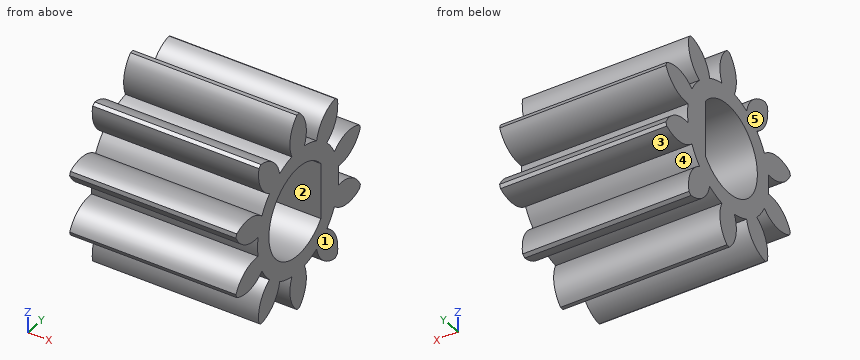
from build123d import *

# Parameters (mm, degrees)
SPUR_START             = -9.526796012
SPUR_GEAR_AM_OUTLINE_R = 2.5
SPUR_GEAR_AM_DEPTH     = 10
SKETCH1_R              = 2.7
CUT_EXTRUDE1_DEPTH     = 14.319939227
BOSS_EXTRUDE1_DEPTH    = 10


# Read off the part's stored shape, not the designer's step: spur gear_am
with BuildPart() as part:
    # spur gear_am outline → spur gear_am (new body)
    with BuildSketch(Plane.YZ.offset(SPUR_START)):
        with BuildLine():
            ThreePointArc((-0.156519062, -5.364277595), (-0.037626451, -5.365455666), (0.081266159, -5.364277595))
            ThreePointArc((0.081266159, -5.364277595), (0.682735226, -4.291319539), (0.542534544, -3.069293435))
            ThreePointArc((0.542534544, -3.069293435), (1.12087826, -2.930966545), (1.670074661, -2.702933442))
            ThreePointArc((1.670074661, -2.702933442), (2.274938849, -3.773981221), (3.392206468, -4.288487876))
            ThreePointArc((3.392206468, -4.288487876), (3.489085062, -4.219557632), (3.584578752, -4.14872123))
            ThreePointArc((3.584578752, -4.14872123), (3.440508527, -2.927145281), (2.608794871, -2.020913288))
            ThreePointArc((2.608794871, -2.020913288), (2.995378261, -1.569062577), (3.305652987, -1.061770376))
            ThreePointArc((3.305652987, -1.061770376), (4.424544483, -1.572735982), (5.630852398, -1.33226718))
            ThreePointArc((5.630852398, -1.33226718), (5.668712646, -1.219557632), (5.704332072, -1.106119996))
            ThreePointArc((5.704332072, -1.106119996), (4.869752484, -0.202526647), (3.664212201, 0.041761415))
            ThreePointArc((3.664212201, 0.041761415), (3.711373549, 0.634544334), (3.664212201, 1.227327254))
            ThreePointArc((3.664212201, 1.227327254), (4.869752484, 1.471615316), (5.704332072, 2.375208665))
            ThreePointArc((5.704332072, 2.375208665), (5.668712646, 2.488646301), (5.630852398, 2.601355849))
            ThreePointArc((5.630852398, 2.601355849), (4.424544483, 2.84182465), (3.305652987, 2.330859045))
            ThreePointArc((3.305652987, 2.330859045), (2.995378261, 2.838151246), (2.608794871, 3.290001957))
            ThreePointArc((2.608794871, 3.290001957), (3.440508527, 4.19623395), (3.584578752, 5.417809899))
            ThreePointArc((3.584578752, 5.417809899), (3.489085062, 5.488646301), (3.392206468, 5.557576545))
            ThreePointArc((3.392206468, 5.557576545), (2.274938849, 5.04306989), (1.670074661, 3.972022111))
            ThreePointArc((1.670074661, 3.972022111), (1.12087826, 4.200055214), (0.542534544, 4.338382103))
            ThreePointArc((0.542534544, 4.338382103), (0.682735226, 5.560408207), (0.081266159, 6.633366264))
            ThreePointArc((0.081266159, 6.633366264), (-0.037626451, 6.634544334), (-0.156519062, 6.633366264))
            ThreePointArc((-0.156519062, 6.633366264), (-0.757988129, 5.560408207), (-0.617787447, 4.338382103))
            ThreePointArc((-0.617787447, 4.338382103), (-1.196131163, 4.200055214), (-1.745327564, 3.972022111))
            ThreePointArc((-1.745327564, 3.972022111), (-2.350191752, 5.04306989), (-3.467459371, 5.557576545))
            ThreePointArc((-3.467459371, 5.557576545), (-3.564337965, 5.488646301), (-3.659831655, 5.417809899))
            ThreePointArc((-3.659831655, 5.417809899), (-3.51576143, 4.19623395), (-2.684047774, 3.290001957))
            ThreePointArc((-2.684047774, 3.290001957), (-3.070631163, 2.838151245), (-3.38090589, 2.330859045))
            ThreePointArc((-3.38090589, 2.330859045), (-4.499797386, 2.84182465), (-5.706105301, 2.601355849))
            ThreePointArc((-5.706105301, 2.601355849), (-5.743965549, 2.488646301), (-5.779584975, 2.375208665))
            ThreePointArc((-5.779584975, 2.375208665), (-4.945005387, 1.471615316), (-3.739465104, 1.227327254))
            ThreePointArc((-3.739465104, 1.227327254), (-3.786626451, 0.634544334), (-3.739465104, 0.041761415))
            ThreePointArc((-3.739465104, 0.041761415), (-4.945005387, -0.202526647), (-5.779584975, -1.106119996))
            ThreePointArc((-5.779584975, -1.106119996), (-5.743965549, -1.219557632), (-5.706105301, -1.33226718))
            ThreePointArc((-5.706105301, -1.33226718), (-4.499797386, -1.572735982), (-3.38090589, -1.061770376))
            ThreePointArc((-3.38090589, -1.061770376), (-3.070631163, -1.569062576), (-2.684047774, -2.020913288))
            ThreePointArc((-2.684047774, -2.020913288), (-3.51576143, -2.927145281), (-3.659831655, -4.14872123))
            ThreePointArc((-3.659831655, -4.14872123), (-3.564337965, -4.219557632), (-3.467459371, -4.288487876))
            ThreePointArc((-3.467459371, -4.288487876), (-2.350191752, -3.773981221), (-1.745327564, -2.702933442))
            ThreePointArc((-1.745327564, -2.702933442), (-1.196131163, -2.930966545), (-0.617787447, -3.069293435))
            ThreePointArc((-0.617787447, -3.069293435), (-0.757988129, -4.291319539), (-0.156519062, -5.364277595))
        make_face()
        with Locations((-0.037626451, 0.634544334)):
            Circle(SPUR_GEAR_AM_OUTLINE_R, mode=Mode.SUBTRACT)
    extrude(amount=SPUR_GEAR_AM_DEPTH)

    # Sketch1 → Cut-Extrude1 (cut, through all)
    with BuildSketch(Plane.ZY.offset(9.526796012)):
        with Locations((0.634544334, -0.037626451)):
            Circle(SKETCH1_R)
    extrude(amount=-CUT_EXTRUDE1_DEPTH, mode=Mode.SUBTRACT)

    # Sketch2 → Boss-Extrude1 (add, through all)
    with BuildSketch(Plane.ZY.offset(9.526796012)):
        with BuildLine():
            Line((2.331600609, 2.062373549), (-1.06251194, 2.062373549))
            ThreePointArc((-1.06251194, 2.062373549), (0.634544334, 2.662373549), (2.331600609, 2.062373549))
        make_face()
    extrude(amount=-BOSS_EXTRUDE1_DEPTH)


solid = part.part
The model under review builds one solid part; all positions refer to its coordinate system, in mm. Face numbers are marked on the shaded views. A direction names the side the tool comes from. Coordinates: 2 decimals unless noted, no trailing zeros. Order: outer loops, then holes, each group sorted by start corner. A loop starts at its lowest first (then second) coordinate and runs counter-clockwise, first axis right, second up. Notation, with made-up numbers: (39, 13) -> (82, 13) arc R26 cw to (82, 28) -> close; hole circle Ø3 at (89.25, 74). An arc over 180 degrees is marked (long way). Answer in a Markdown table with one row per item.
(1) Consider section B-B (y = -4.5). Write out the cut boundary in (x, z).
Answers:
| item | result |
|---|---|
| outline | (-9.53, -1.57) -> (0.47, -1.57) -> (0.47, -0.02) -> (-9.53, -0.02) -> close; (-9.53, 1.29) -> (0.47, 1.29) -> (0.47, 2.84) -> (-9.53, 2.84) -> close |
(2) The part is to be moulded in two halves that separate along Y. For the marked faces 3, 4 and 5, say which applies: +Y half, -Y half, draft (parallel to the pull), parting line (faces both ways), or undercut.
Answers:
| item | result |
|---|---|
| face 3 | undercut |
| face 4 | undercut |
| face 5 | draft |
(3) Consider section D-D (z = -2.25). Write out the cut boundary in (x, y).
Answers:
| item | result |
|---|---|
| outline | (-9.53, -3.01) -> (0.47, -3.01) -> (0.47, 2.93) -> (-9.53, 2.93) -> close |
(4) Insertion check: pin 1 (1.7 mm diameter, centred on x = -4.5, z = 0.5, fed in from -Y); pin 2 (6 mm diameter, centred on x = -1.5, y = -4, fed in from -Z); pin 3 (6 mm diameter, centred on x = -5, y = 3.5, fed in from +Z). Each pin has a flat end and moves straight along its axis. Give the tip position at first contact, or say it passes through.
Answers:
| item | result |
|---|---|
| pin 1 | y = -5.17 |
| pin 2 | z = -4.29 |
| pin 3 | z = 6.08 |
(5) Consider section C-C (z = 0.5). Write out the cut boundary in (x, y), plus the area to 3 significant figures.
Answers:
| item | result |
|---|---|
| outline | (-9.53, -3.78) -> (0.47, -3.78) -> (0.47, -2.73) -> (-9.53, -2.73) -> close; (-9.53, 2.06) -> (0.47, 2.06) -> (0.47, 3.71) -> (-9.53, 3.71) -> close |
| area | 27.0 mm² |
(6) Consider section A-A (z = -3.5). Write out the cut boundary in (x, y).
Answers:
| item | result |
|---|---|
| outline | (-9.53, -3.68) -> (0.47, -3.68) -> (0.47, -2.1) -> (-9.53, -2.1) -> close; (-9.53, -0.76) -> (0.47, -0.76) -> (0.47, 0.68) -> (-9.53, 0.68) -> close; (-9.53, 2.03) -> (0.47, 2.03) -> (0.47, 3.61) -> (-9.53, 3.61) -> close |
(7) Machinability: for the marked faces 1 and 2, which of the approach directions +Z, -Z, +X, -X, +Y, -Y give a long, thin tool a straight path to every point of the face, cutting with its end or side? Answer none if there is none.
Answers:
| item | result |
|---|---|
| face 1 | +Z, -Z, +X, +Y, -Y |
| face 2 | +X, -X |
(8) Wall thickness on line 1 along Y through (x, z) = (-0.25, 0.75); line 2 along Y through (x, z) = (-4, 5.25); line 3 along Y through (x, z) = (-8.25, -3.5): over which ranges is each line inside the solid? List them lowest first.
Answers:
| item | result |
|---|---|
| line 1 | -3.78 to -2.74, 2.06 to 3.71 |
| line 2 | -3.69 to -2.62, -0.8 to 0.72, 2.54 to 3.61 |
| line 3 | -3.68 to -2.1, -0.76 to 0.68, 2.03 to 3.61 |
